from build123d import *

# Parameters (mm, degrees)
SKETCH1_W           = 127.76
SKETCH1_H           = 85.48
BOSS_EXTRUDE1_DEPTH = 20
CUT_EXTRUDE1_START  = -5
CUT_EXTRUDE1_DEPTH  = 20


with BuildPart() as part:
    # Sketch1 → Boss-Extrude1 (new body)
    with BuildSketch(Plane(origin=(0, 0, 0), x_dir=(1, 0, 0), z_dir=(0, 1, 0))):
        with Locations((63.88, 42.74)):
            Rectangle(SKETCH1_W, SKETCH1_H)
    extrude(amount=BOSS_EXTRUDE1_DEPTH)

    # Sketch2 → Cut-Extrude1 (cut)
    with BuildSketch(Plane(origin=(0, 20, 0), x_dir=(1, 0, 0), z_dir=(0, 1, 0)).offset(CUT_EXTRUDE1_START)):
        Polygon((76.96, 85.48), (50.8, 85.48), (50.8, 12.7), (50.8, 0), (76.96, 0), (76.96, 72.78), align=None)
    extrude(amount=-CUT_EXTRUDE1_DEPTH, mode=Mode.SUBTRACT)


solid = part.part
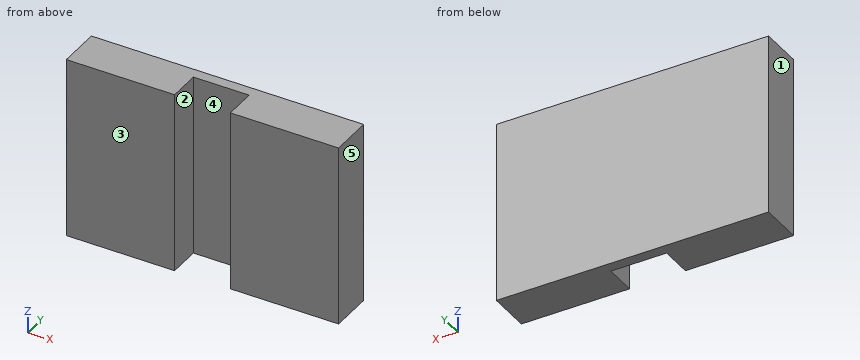
Read the model definition and answer for the solid it produces. Units are mm, in the model's axes. Face numbers are marked on the shaded views. A direction names the side the tool comes from. Give positions to 0.01 mm unless a question says otherwise; leave off trailing zeros. Loops run counter-clockwise (first coordinate to the right, second up) from the corner with the lowest first, then second, coordinate; pieces in that order, holes last. Notation, with made-up numbers: (-37.75, 54.25) -> (-29.75, 54.25) arc R17 cw to (-29.75, 63.25) -> close; hole circle Ø5 at (27, 62.25). An arc over 180 degrees is marked (long way). Answer as CSV lines item,"result".
Item 1: Determine the mould class of the marked faces 1, 2 and 3 for opening direction X: +X half, -X half, draft (parallel to the pull), parting line (faces both ways), or undercut.
Returned:
face 1,"-X half"
face 2,"undercut"
face 3,"draft"
Item 2: Consider line 1 (X direction, y = 1.5, z = -12); line 2 (Y direction, x = 58.5, z = -38.5). Determine where each line is inside the solid, lowest interval first. Write a range as [from, to].
Returned:
line 1,"x = [0, 50.8], [76.96, 127.76]"
line 2,"y = [15, 20]"
Item 3: Each of these flat-tipped pins is pushed along its axis until it touches: pin 1 (2 mm diameter, centred on y = 7.5, z = -28.5, fed in from -X); pin 2 (13 mm diameter, centred on x = 62, z = -33.5, fed in from -Y). Where does it stop, or does it pass through?
Returned:
pin 1,"stops at x = 0"
pin 2,"stops at y = 15"
Item 4: Find section B-B on z = -47. Give the vertices of the cut face in (x, y), plus the area to 3 significant figures.
Returned:
outline,"(0, 0) -> (50.8, 0) -> (50.8, 15) -> (76.96, 15) -> (76.96, 0) -> (127.76, 0) -> (127.76, 20) -> (0, 20) -> close"
area,"2,160 mm²"
Item 5: Find section C-C on x = 67. Give the vertices of the cut face in (y, z), plus the area to 3 significant figures.
Returned:
outline,"(15, -85.48) -> (20, -85.48) -> (20, 0) -> (15, 0) -> close"
area,"427 mm²"
Item 6: For the marked faces 4 and 5, determine the directions among +Z, -Z, +X, -X, +Y, -Y from which every point of the face is accessible in a straight line to the end or side of a thin tool.
Returned:
face 4,"+Z, -Z, -Y"
face 5,"+Z, -Z, +X, +Y, -Y"
Item 7: Find section A-A on y = 2. Give the vertices of the cut face in (x, z).
Returned:
outline,"(0, -85.48) -> (50.8, -85.48) -> (50.8, 0) -> (0, 0) -> close; (76.96, -85.48) -> (127.76, -85.48) -> (127.76, 0) -> (76.96, 0) -> close"
